Design review of the part built by this model. Coordinates are the model's own, in mm. Face numbers are marked on the shaded views. A direction names the side the tool comes from. Round coordinates to 2 decimals unless told otherwise and drop trailing zeros. Loops run counter-clockwise (first coordinate to the right, second up) from the corner with the lowest first, then second, coordinate; pieces in that order, holes last. Notation, with made-up numbers: M 68,-3.5 L 83,-3.5 A17 ccw 83,27.5 Z; hole C 7,60.25 d8. An arc over 180 degrees is marked long. One line per item, written item: value. Start each with the question number.
Item 1: For the marked faces 4, 5, 6 and 7, list the 3-axis set-ups (+Z, -Z, +X, -X, +Y, -Y) from which the entire face can be reached by the end or side of a thin tool; tool diameter is ignored.
Item 2: Mouldability with a two-part tool opening along Y and no side actions: class the marked faces 1, 2 and 3 as released by +Y, released by -Y, zero draft, split by the parting line, or undercut.
Item 3: We need section B-B (x = 0). Write out the cut boundary in (y, z), then the cut area to 3 significant figures.
Item 4: We need section C-C (z = 5.5). Write out the cut boundary in (x, y), then the cut area to 3 significant figures.
Item 5: For line 1 along Y through (x, z) = (2.75, -13.25); line 2 along X through (y, z) = (2, -1.75); line 3 along Y through (x, z) = (2.5, -8.25), list the stretches that pass through material, from the lowest coordinate up.
Item 6: We need section A-A (y = 6.25). Write out the cut boundary in (x, z).
Item 7: Clearance check with flat-ended pins moving along their axes: pin 1 (3 mm diameter, centred on x = -9, y = 3, fed in from -Z); pin 2 (3 mm diameter, centred on y = 6, z = -11, fed in from +X); pin 3 (3 mm diameter, centred on y = 8.5, z = -11.5, fed in from +X). State where each tip first meets the part, or that it passes through.
Item 8: We need section D-D (y = 0.5). Write out the cut boundary in (x, z), then the cut area to 3 significant figures.
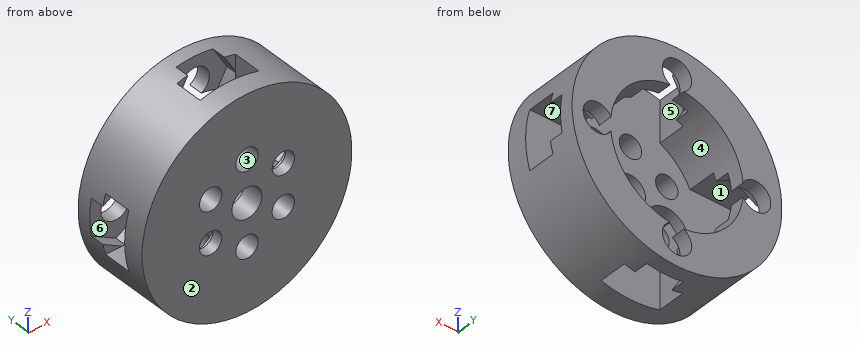
from build123d import *

# Parameters (mm, degrees)
SKETCH1_R           = 10
SKETCH1_R_2         = 1.6
SKETCH1_R_3         = 2.15
BOSS_EXTRUDE1_DEPTH = 3
SKETCH2_R           = 3.1
CUT_EXTRUDE2_DEPTH  = 1.5
SKETCH3_R           = 15
SKETCH3_R_2         = 9.5
BOSS_EXTRUDE2_DEPTH = 11
SKETCH5_R           = 2.1
CUT_EXTRUDE3_DEPTH  = 4
SKETCH7_W           = 10
SKETCH7_H           = 8.4
SKETCH7_W_2         = 8.4
SKETCH7_H_2         = 10
CUT_EXTRUDE4_DEPTH  = 4
CUT_EXTRUDE6_DEPTH  = 2


with BuildPart() as part:
    # Sketch1 → Boss-Extrude1 (new body)
    with BuildSketch(Plane(origin=(0, 0, 0), x_dir=(1, 0, 0), z_dir=(0, 1, 0))):
        with Locations(Location((0, 0, 0), (0, 0, 270))):
            Circle(SKETCH1_R)
        with Locations(Location((0, 6, 0), (0, 0, 270))):
            Circle(SKETCH1_R_2, mode=Mode.SUBTRACT)
        with Locations(Location((5.196152423, 3, 0), (0, 0, 270))):
            Circle(SKETCH1_R_2, mode=Mode.SUBTRACT)
        with Locations(Location((5.196152423, -3, 0), (0, 0, 270))):
            Circle(SKETCH1_R_2, mode=Mode.SUBTRACT)
        with Locations(Location((0, -6, 0), (0, 0, 270))):
            Circle(SKETCH1_R_2, mode=Mode.SUBTRACT)
        with Locations(Location((-5.196152423, -3, 0), (0, 0, 270))):
            Circle(SKETCH1_R_2, mode=Mode.SUBTRACT)
        with Locations(Location((-5.196152423, 3, 0), (0, 0, 270))):
            Circle(SKETCH1_R_2, mode=Mode.SUBTRACT)
        with Locations(Location((0, 0, 0), (0, 0, 270))):
            Circle(SKETCH1_R_3, mode=Mode.SUBTRACT)
    extrude(amount=BOSS_EXTRUDE1_DEPTH)

    # Sketch2 → Cut-Extrude2 (cut)
    with BuildSketch(Plane(origin=(0, 3, 0), x_dir=(1, 0, 0), z_dir=(0, 1, 0))):
        with Locations(Location((-5.196152423, 3, 0), (0, 0, 270))):
            Circle(SKETCH2_R)
        with Locations(Location((5.196152423, -3, 0), (0, 0, 270))):
            Circle(SKETCH2_R)
    extrude(amount=-CUT_EXTRUDE2_DEPTH, mode=Mode.SUBTRACT)

    # Sketch3 → Boss-Extrude2 (add)
    with BuildSketch(Plane.XZ):
        with Locations(Location((0, 0, 0), (0, 0, 270))):
            Circle(SKETCH3_R)
        with Locations(Location((0, 0, 0), (0, 0, 270))):
            Circle(SKETCH3_R_2, mode=Mode.SUBTRACT)
    extrude(amount=-BOSS_EXTRUDE2_DEPTH)

    # Sketch5 → Cut-Extrude3 (cut)
    with BuildSketch(Plane(origin=(0, 11, 0), x_dir=(1, 0, 0), z_dir=(0, 1, 0))):
        with Locations((0, 11.313708499)):
            Circle(SKETCH5_R)
        with Locations((11.313708499, 0)):
            Circle(SKETCH5_R)
        with Locations((0, -11.313708499)):
            Circle(SKETCH5_R)
        with Locations((-11.313708499, 0)):
            Circle(SKETCH5_R)
    extrude(amount=-CUT_EXTRUDE3_DEPTH, mode=Mode.SUBTRACT)

    # Sketch7 → Cut-Extrude4 (cut)
    with BuildSketch(Plane(origin=(0, 7, 0), x_dir=(1, 0, 0), z_dir=(0, 1, 0))):
        with Locations((-12.313708499, 0)):
            Rectangle(SKETCH7_W, SKETCH7_H)
        with Locations((0, 12.313708499)):
            Rectangle(SKETCH7_W_2, SKETCH7_H_2)
        with Locations((12.313708499, 0)):
            Rectangle(SKETCH7_W, SKETCH7_H)
        with Locations((0, -12.313708499)):
            Rectangle(SKETCH7_W_2, SKETCH7_H_2)
    extrude(amount=-CUT_EXTRUDE4_DEPTH, mode=Mode.SUBTRACT)

    # Sketch8 → Cut-Extrude6 (cut)
    with BuildSketch(Plane.XZ.offset(-7)):
        Polygon((-2.257631932, 7.284262955), (2.360786238, 7.343819121), (4.61841817, 11.373264666), (2.257631932, 15.343154043), (-2.360786238, 15.283597877), (-4.61841817, 11.254152332), align=None)
        Polygon((-7.284262955, -2.257631932), (-7.343819121, 2.360786238), (-11.373264666, 4.61841817), (-15.343154043, 2.257631932), (-15.283597877, -2.360786238), (-11.254152332, -4.61841817), align=None)
        Polygon((7.284262955, 2.257631932), (7.343819121, -2.360786238), (11.373264666, -4.61841817), (15.343154043, -2.257631932), (15.283597877, 2.360786238), (11.254152332, 4.61841817), align=None)
        Polygon((2.257631932, -7.284262955), (-2.360786238, -7.343819121), (-4.61841817, -11.373264666), (-2.257631932, -15.343154043), (2.360786238, -15.283597877), (4.61841817, -11.254152332), align=None)
    extrude(amount=-CUT_EXTRUDE6_DEPTH, mode=Mode.SUBTRACT)


solid = part.part
A:
1. face 4: +Y
1. face 5: +Z, -Z
1. face 6: none
1. face 7: +X, -X
2. face 1: undercut
2. face 2: released by -Y
2. face 3: zero draft
3. outline: M 0,-15 L 3,-15 L 3,-7.6 L 0,-7.6 Z; M 0,-4.4 L 3,-4.4 L 3,-2.15 L 0,-2.15 Z; M 0,2.15 L 3,2.15 L 3,4.4 L 0,4.4 Z; M 0,7.6 L 3,7.6 L 3,15 L 0,15 Z; M 9,-15 L 11,-15 L 11,-13.41 L 9,-13.41 Z; M 9,13.41 L 11,13.41 L 11,15 L 9,15 Z
3. area: 64.2 mm2
4. outline: M -13.96,0 L -1.52,0 L -1.52,3 L -7.75,3 L -7.75,11 L -13.96,11 Z; M 1.52,0 L 13.96,0 L 13.96,11 L 7.75,11 L 7.75,3 L 7.03,3 L 7.03,1.5 L 3.36,1.5 L 3.36,3 L 1.52,3 Z
4. area: 168 mm2
5. line 1: 0 to 3, 9 to 11
5. line 2: -14.9 to -8.03, -2.36 to -1.25, 1.25 to 4.2, 6.19 to 14.9
5. line 3: 0 to 3
6. outline: M -14.4,-4.2 A15 ccw -4.2,-14.4 L -4.2,-8.52 A9.5 cw -8.52,-4.2 Z; M -14.4,4.2 L -8.52,4.2 A9.5 cw -4.2,8.52 L -4.2,14.4 A15 ccw Z; M 4.2,-14.4 A15 ccw 14.4,-4.2 L 8.52,-4.2 A9.5 cw 4.2,-8.52 Z; M 4.2,8.52 A9.5 cw 8.52,4.2 L 14.4,4.2 A15 ccw 4.2,14.4 Z
7. pin 1: z = -12.99
7. pin 2: x = 11.61
7. pin 3: x = 11.18
8. outline: C 0,0 d30; hole C -5.2,-3 d3.2; hole C -5.2,3 d3.2; hole C 0,0 d4.3; hole C 0,-6 d3.2; hole C 0,6 d3.2; hole C 5.2,-3 d3.2; hole C 5.2,3 d3.2
8. area: 644 mm2
